Part print with two shaded views. Sizes in mm from the minimum x, y, z corner. A direction names the side the tool comes from. Give positions to 0.01 mm unless a question says otherwise; leave off trailing zeros. Write each loop counter-clockwise with the first axis right and the second up, starting at its lowest first coordinate (ties: lowest second). Pieces come first, ordered by that corner, then holes. Notation, with made-up numbers: (-33, 17.25) - (17, 17.25) arc R26 cw to (17, 52.25) - close; hole circle Ø1 at (67.5, 6). An arc over 180 degrees is marked (long way). One line per item, written item: value. Start each with the question number.
(1) Cut at A-A, the plane z = 121. List the corners of the cut face in (x, y).
(2) 3-axis set-ups, long thin cutter, end or side, ignore diameter. For the marked faces 1 and 2: which of +Z, -Z, +X, -X, +Y, -Y reach the whole face in a straight line?
(3) Cut at B-B, the plane y = 99.5. List the corners of the cut face in (x, z).
(4) Cut at C-C, the plane x = 184.5. List the corners of the cut face in (y, z), and give its area (3 significant figures).
(5) Probe L1, parallel to X at y = 25.5, z = 46.5; L2, parallel to Z at x = 53, y = 70.5; L3, parallel to X at y = 98.5, z = 140. List the from-to ranges inside material, lowest first.
(6) Cut at D-D, the plane x = 116. List the corners of the cut face in (y, z), and give its area (3 significant figures).
(7) Drop a flat-ended pin along its axis: P1, Ø12, axis at x = 51, z = 140, coming from the +Y side. Give the stop position or say it passes through.
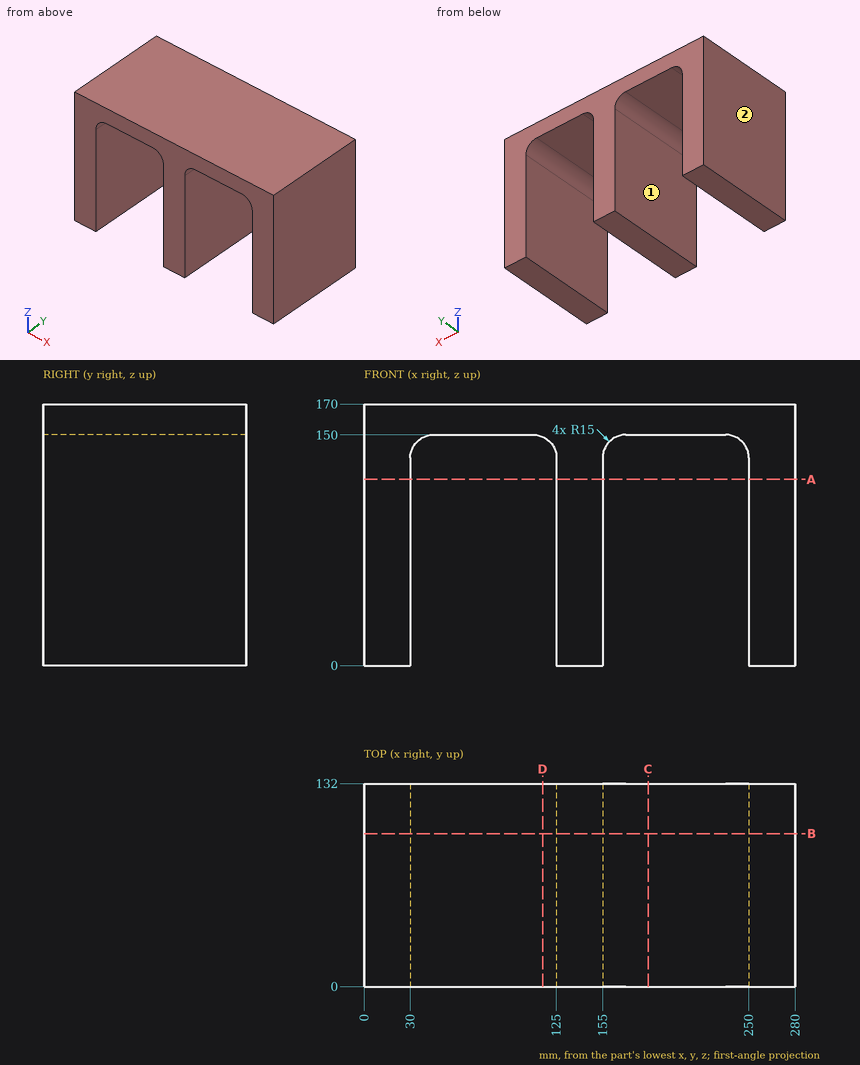
Answers follow:
1. outline: (0, 0) - (30, 0) - (30, 132) - (0, 132) - close; (125, 0) - (155, 0) - (155, 132) - (125, 132) - close; (250, 0) - (280, 0) - (280, 132) - (250, 132) - close
2. face 1: -Z, +Y, -Y
2. face 2: +Z, -Z, -X, +Y, -Y
3. outline: (0, 0) - (30, 0) - (30, 135) arc R15 cw to (45, 150) - (110, 150) arc R15 cw to (125, 135) - (125, 0) - (155, 0) - (155, 135) arc R15 cw to (170, 150) - (235, 150) arc R15 cw to (250, 135) - (250, 0) - (280, 0) - (280, 170) - (0, 170) - close
4. outline: (0, 150) - (132, 150) - (132, 170) - (0, 170) - close
4. area: 2,640 mm²
5. L1: x = 0 to 30, 125 to 155, 250 to 280
5. L2: z = 150 to 170
5. L3: x = 0 to 30.86, 124.14 to 155.86, 249.14 to 280
6. outline: (0, 148.75) - (132, 148.75) - (132, 170) - (0, 170) - close
6. area: 2,810 mm²
7. P1: passes through
